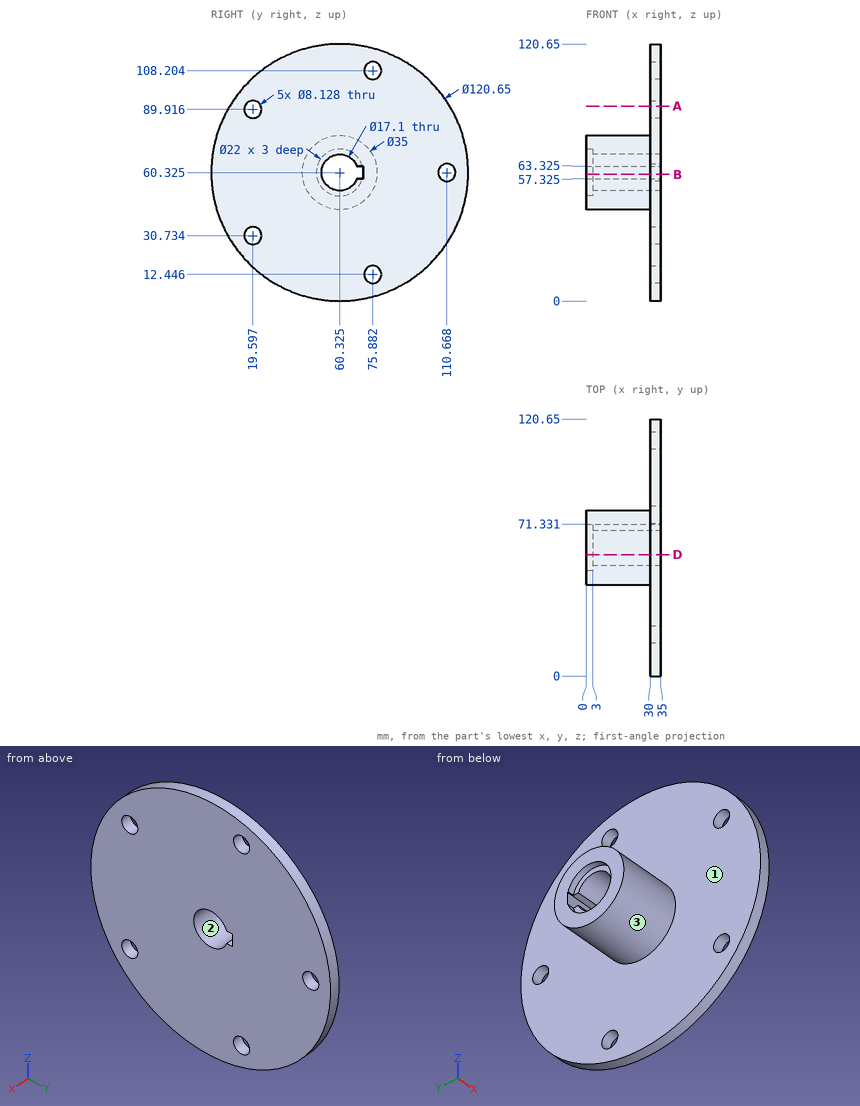
Can you work these out from the drawing? Everything is in mm from the part's minimum corner. Give positions to 0.01 mm unless a question says otherwise; leave off trailing zeros. Order: outer loops, then holes, each group sorted by start corner. A loop starts at its lowest first (then second) coordinate and runs counter-clockwise, first axis right, second up.
1. We'd pull the mould along Y, two halves only. Please class the marked faces 1, 2 and 3: pulls with the +Y half, pulls with the -Y half, needs draft (parallel to the pull), parting line crosses it, or undercut.
2. Suppose I cut it at B-B (z = 59.5). List the corners of the cut face in (x, y) for me (1 decimal).
3. Suppose I cut it at D-D (y = 57). List the corners of the cut face in (x, z) for me, plus the area to 3 significant figures.
4. Suppose I cut it at A-A (z = 91.5). List the corners of the cut face in (x, y) for me.
5. I need wall thicknesses on L1, parallel to X at y = 76, z = 115; L2, parallel to Y at x = 18, z = 67.5 (1 decimal); L3, parallel to Z at x = 11.5, y = 56.5. Which ranges of each line are inside material? Lowest first, please.
6. Will these pins go through, and if not, where does the flat tip stop? P1, Ø5, axis at y = 19.6, z = 30.73, coming from the +X side; P2, Ø0.9, axis at x = 17.5, y = 70, coming from the +Z side (1 decimal); P3, Ø10.5, axis at y = 75.88, z = 12.45, coming from the +X side; P4, Ø9.5, axis at y = 75.88, z = 108.2, coming from the -X side.
Solved:
1. face 1: needs draft
1. face 2: undercut
1. face 3: parting line crosses it
2. outline: (0, 42.8) - (30, 42.8) - (30, 0) - (35, 0) - (35, 51.8) - (3, 51.8) - (3, 49.4) - (0, 49.4) - close; (0, 71.3) - (35, 71.3) - (35, 106.7) - (30, 106.7) - (30, 77.8) - (0, 77.8) - close; (30, 114.6) - (35, 114.6) - (35, 120.6) - (30, 120.6) - close
3. outline: (0, 43.14) - (30, 43.14) - (30, 0.09) - (35, 0.09) - (35, 52.45) - (3, 52.45) - (3, 49.84) - (0, 49.84) - close; (0, 70.81) - (3, 70.81) - (3, 68.2) - (35, 68.2) - (35, 120.56) - (30, 120.56) - (30, 77.51) - (0, 77.51) - close
3. area: 1,070 mm2
4. outline: (30, 8.68) - (35, 8.68) - (35, 15.85) - (30, 15.85) - close; (30, 23.34) - (35, 23.34) - (35, 111.97) - (30, 111.97) - close
5. L1: x = 30 to 35
5. L2: y = 44.4 to 55.7, 65 to 76.3
5. L3: z = 43.25 to 52.68, 67.97 to 77.4
6. P1: passes through
6. P2: stops at z = 75.2
6. P3: stops at x = 35
6. P4: stops at x = 30
